Verification items for the finished model (mm, model axes). Face numbers are marked on the shaded views. Round coordinates to 2 decimals unless told otherwise and drop trailing zeros. Write each loop counter-clockwise with the first axis right and the second up, starting at its lowest first coordinate (ties: lowest second). Pieces come first, ordered by that corner, then holes.
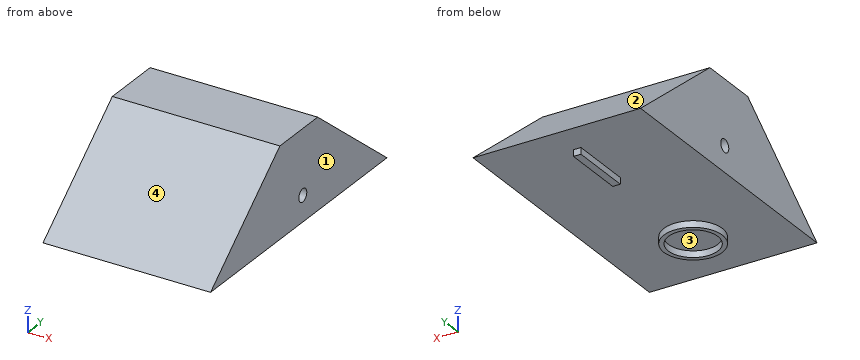
from build123d import *

# Parameters (mm, degrees)
IZIM1_W                     = 13
IZIM1_H                     = 22
Y_KSEKLIK_EKSTR_ZYON1_DEPTH = 7
KES_EKSTR_ZYON1_DEPTH       = 19.41195264
IZIM3_W                     = 0.583664442
IZIM3_H                     = 4.902781318
IZIM3_R                     = 2.271047272
Y_KSEKLIK_EKSTR_ZYON2_DEPTH = 0.5
IZIM4_R                     = 1.923937322
KES_EKSTR_ZYON2_DEPTH       = 0.5
IZIM5_R                     = 0.5
KES_EKSTR_ZYON3_DEPTH       = 19.41195264


with BuildPart() as part:
    # Çizim1 → Yükseklik-Ekstrüzyon1 (new body)
    with BuildSketch(Plane.XY):
        Rectangle(IZIM1_W, IZIM1_H)
    extrude(amount=Y_KSEKLIK_EKSTR_ZYON1_DEPTH)

    # Çizim2 → Kes-Ekstrüzyon1 (cut, through all)
    with BuildSketch(Plane(origin=(6.5, 0, 0), x_dir=(0, 0, -1), z_dir=(1, 0, 0))):
        Polygon((-7, 2.355719904), (0, 11), (-7, 11), align=None)
        Polygon((0, -11), (-7, -2.355719904), (-7, -11), align=None)
    extrude(amount=-KES_EKSTR_ZYON1_DEPTH, mode=Mode.SUBTRACT)

    # Çizim3 → Yükseklik-Ekstrüzyon2 (add)
    with BuildSketch(Plane(origin=(0, 0, 0), x_dir=(-1, 0, 0), z_dir=(0, 0, -1))):
        with Locations((0, 6)):
            Rectangle(IZIM3_W, IZIM3_H)
        with Locations(Location((0, -6, 0), (0, 0, 180))):
            Circle(IZIM3_R)
    extrude(amount=Y_KSEKLIK_EKSTR_ZYON2_DEPTH)

    # Çizim4 → Kes-Ekstrüzyon2 (cut)
    with BuildSketch(Plane(origin=(0, 0, -0.5), x_dir=(-1, 0, 0), z_dir=(0, 0, -1))):
        with Locations((0, -6)):
            Circle(IZIM4_R)
    extrude(amount=-KES_EKSTR_ZYON2_DEPTH, mode=Mode.SUBTRACT)

    # Çizim5 → Kes-Ekstrüzyon3 (cut, through all)
    with BuildSketch(Plane(origin=(6.5, 0, 0), x_dir=(0, 0, -1), z_dir=(1, 0, 0))):
        with Locations(Location((-2, 0.5, 0), (0, 0, 90))):
            Circle(IZIM5_R)
    extrude(amount=-KES_EKSTR_ZYON3_DEPTH, mode=Mode.SUBTRACT)


solid = part.part
Q1. Material ranges on line 1 along Y through (x, z) = (0, -0.3); line 2 along Z through (x, y) = (3, 0.5); line 3 along Z through (x, y) = (-0.5, -2.25), recorded low to high.
Recorded:
line 1: y = -8.27 to -7.92, -4.08 to -3.73, 3.55 to 8.45
line 2: z = 0 to 1.5, 2.5 to 7
line 3: z = 0 to 7
Q2. Sectioned sample at D-D (x = 0). Enter the section's corners in (y, z), plus the area to 3 significant figures.
Recorded:
outline: (-11, 0) - (-8.27, 0) - (-8.27, -0.5) - (-7.92, -0.5) - (-7.92, 0) - (-4.08, 0) - (-4.08, -0.5) - (-3.73, -0.5) - (-3.73, 0) - (3.55, 0) - (3.55, -0.5) - (8.45, -0.5) - (8.45, 0) - (11, 0) - (2.36, 7) - (-2.36, 7) - close; hole circle Ø1 at (0.5, 2)
area: 95.5 mm2
Q3. Sectioned sample at C-C (z = 1.75). Enter the section's corners in (x, y).
Recorded:
outline: (-6.5, -8.84) - (6.5, -8.84) - (6.5, 0.07) - (-6.5, 0.07) - close; (-6.5, 0.93) - (6.5, 0.93) - (6.5, 8.84) - (-6.5, 8.84) - close
Q4. Sectioned sample at A-A (x = 3). Enter the section's corners in (y, z).
Recorded:
outline: (-11, 0) - (11, 0) - (2.36, 7) - (-2.36, 7) - close; hole circle Ø1 at (0.5, 2)
Q5. Sectioned sample at B-B (y = 0.5). Enter the section's corners in (x, z), plus the area to 3 significant figures.
Recorded:
outline: (-6.5, 0) - (6.5, 0) - (6.5, 1.5) - (-6.5, 1.5) - close; (-6.5, 2.5) - (6.5, 2.5) - (6.5, 7) - (-6.5, 7) - close
area: 78.0 mm2
Q6. Depth check by flat-ended pin: P1, Ø5, axis at x = -3, y = -1.5, coming from the -Z side; P2, Ø4, axis at x = 0.5, y = -6.5, coming from the -Z side; P3, Ø1.5, axis at x = 0, z = 4, coming from the -Y side; P4, Ø3, axis at x = -2.5, z = 2.5, coming from the +Y side. Enter the tip coordinate at first touch or a pass-through.
Recorded:
P1: stops at z = 0
P2: stops at z = -0.5
P3: stops at y = -6.99
P4: stops at y = 9.77
Q7. Release check for a two-part mould opening along Y. For the marked faces 1, 2, 3 and 4 record: released by +Y, released by -Y, zero draft, split by the parting line, or undercut.
Recorded:
face 1: zero draft
face 2: released by +Y
face 3: undercut
face 4: released by -Y
